For this review, use the dimensioned drawing (mm, ordinates from the lowest corner) and the shaded views. Give positions to 0.01 mm unless a question says otherwise; leave off trailing zeros. Order: outer loops, then holes, each group sorted by start corner. A loop starts at its lowest first (then second) coordinate and runs counter-clockwise, first axis right, second up. Notation, with made-up numbers: (1, 41.25) - (28, 41.25) arc R22 ccw to (28, 64.25) - close; hole circle Ø6 at (-29.5, -13.5). An arc over 180 degrees is marked (long way). Use a Markdown table: item, result. Add a question column.
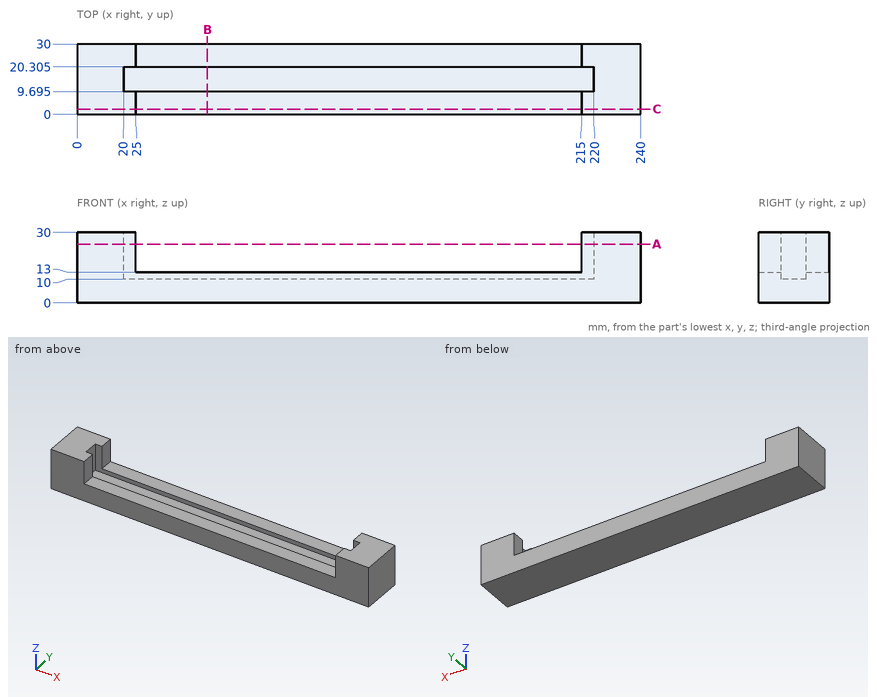
Q1. We need section B-B (x = 55.5). Write out the cut boundary in (y, z) (1 decimal), plus the area to 3 significant figures.
Q2. We need section A-A (z = 25). Write out the cut boundary in (x, y) (1 decimal).
Q3. Clearance check with flat-ended pins moving along their axes: P1, Ø10.5, axis at y = 5.5, z = 22.5, coming from the -X side; P2, Ø3, axis at x = 164.5, y = 15.5, coming from the +Z side; P3, Ø8, axis at x = 166.5, y = 5.5, coming from the +Z side; P4, Ø10, axis at x = 87, z = 20, coming from the -Y side. State where each tip first meets the part, or that it passes through.
Q4. Wall thickness on probe 1 along X at (y, z) = (27.25, 26); probe 2 along X at (y, z) = (19.5, 22.5); probe 3 along Y at (x, z) = (21, 25.75) (1 decimal): over which ranges is each line inside the solid? List them lowest first.
Q5. We need section C-C (y = 2.25). Write out the cut boundary in (x, z).
Here are the results:
| question | item | result |
|---|---|---|
| 1 | outline | (0, 0) - (30, 0) - (30, 13) - (20.3, 13) - (20.3, 10) - (9.7, 10) - (9.7, 13) - (0, 13) - close |
| 1 | area | 358 mm2 |
| 2 | outline | (0, 0) - (25, 0) - (25, 9.7) - (20, 9.7) - (20, 20.3) - (25, 20.3) - (25, 30) - (0, 30) - close; (215, 0) - (240, 0) - (240, 30) - (215, 30) - (215, 20.3) - (220, 20.3) - (220, 9.7) - (215, 9.7) - close |
| 3 | P1 | x = 0 |
| 3 | P2 | z = 10 |
| 3 | P3 | z = 13 |
| 3 | P4 | through |
| 4 | probe 1 | 0 to 25, 215 to 240 |
| 4 | probe 2 | 0 to 20, 220 to 240 |
| 4 | probe 3 | 0 to 9.7, 20.3 to 30 |
| 5 | outline | (0, 0) - (240, 0) - (240, 30) - (215, 30) - (215, 13) - (25, 13) - (25, 30) - (0, 30) - close |
